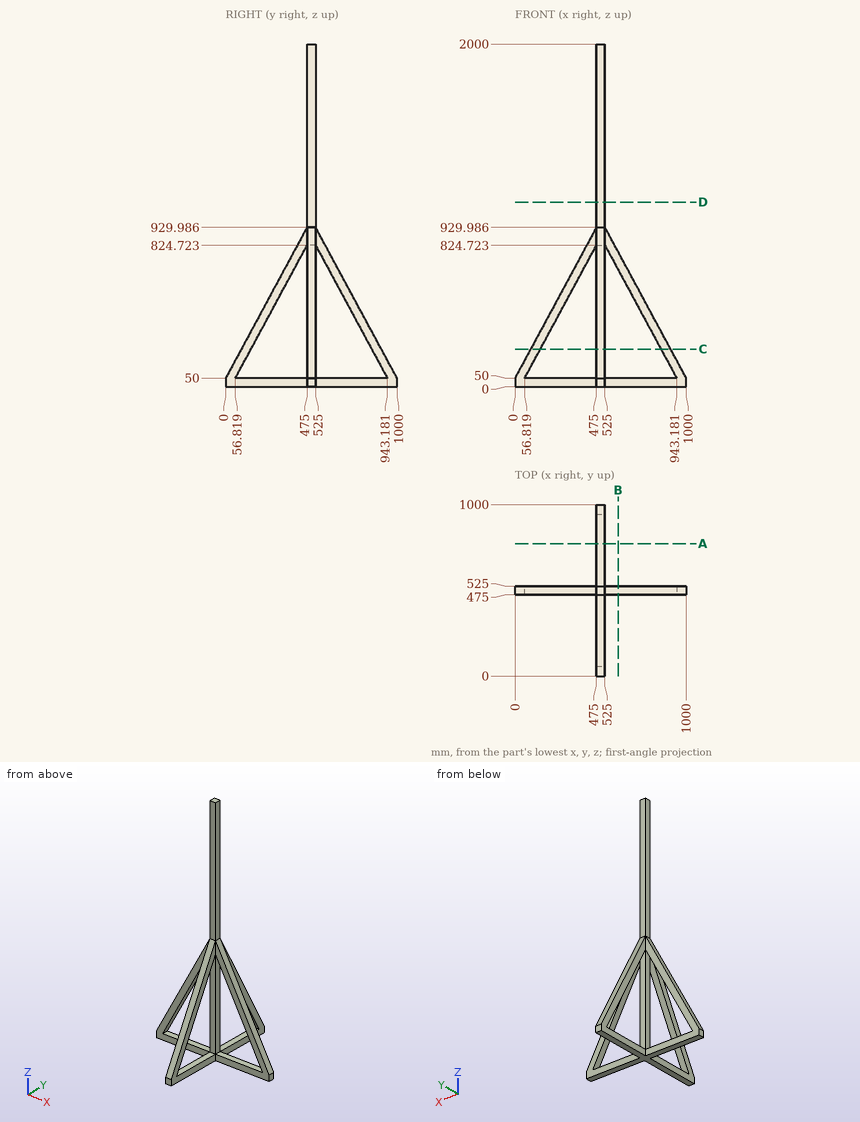
For this review, use the dimensioned drawing (mm, ordinates from the lowest corner) and the shaded views. Coordinates: 2 decimals unless noted, no trailing zeros. Write each loop counter-clockwise with the first axis right and the second up, starting at its lowest first coordinate (ties: lowest second). Pieces come first, ordered by that corner, then holes. Notation, with made-up numbers: (-34, 45.5) - (16, 45.5) arc R28 ccw to (16, 64.5) - close; hole circle Ø11 at (-9, -26.75). An arc over 180 degrees is marked (long way). Answer in a Markdown table with one row per item. Add a question column.
Q1. Consider section D-D on z = 1077.5. Give the boundary of the cut face in (x, y), then the cut area to 3 significant figures.
Q2. Clearance check with flat-ended pins moving along their axes: pin 1 (1 mm diameter, centred on y = 285.5, z = 530.5, fed in from -X); pin 2 (15 mm diameter, centred on x = 508.5, y = 648, fed in from +Z); pin 3 (15 mm diameter, centred on x = 498.5, z = 532, fed in from -Y). State where each tip first meets the part, or that it passes through.
Q3. Consider section C-C on z = 219. Give the boundary of the cut face in (x, y), then the cut area to 3 significant figures.
Q4. Consider section A-A on y = 772. Give the boundary of the cut face in (x, z).
Q5. To check wall thickness, follow line 1 along Y through (x, z) = (647, 693.5); line 2 along Z through (x, y) = (485, 855.5) (1 decimal). State the ranges of each line that lie inside material, in increasing order. Write a range as from..to.
Q6. Consider section B-B on x = 602. Give the boundary of the cut face in (y, z) (1 decimal).
Answers below:
| question | item | result |
|---|---|---|
| 1 | outline | (475, 475) - (525, 475) - (525, 525) - (475, 525) - close |
| 1 | area | 2,500 mm² |
| 2 | pin 1 | x = 475 |
| 2 | pin 2 | z = 716.01 |
| 2 | pin 3 | y = 256.13 |
| 3 | outline | (91.22, 475) - (148.04, 475) - (148.04, 525) - (91.22, 525) - close; (475, 91.22) - (525, 91.22) - (525, 148.04) - (475, 148.04) - close; (475, 475) - (525, 475) - (525, 525) - (475, 525) - close; (475, 851.96) - (525, 851.96) - (525, 908.78) - (475, 908.78) - close; (851.96, 475) - (908.78, 475) - (908.78, 525) - (851.96, 525) - close |
| 3 | area | 13,900 mm² |
| 4 | outline | (475, 0) - (525, 0) - (525, 50) - (475, 50) - close; (475, 367.13) - (525, 367.13) - (525, 472.39) - (475, 472.39) - close |
| 5 | line 1 | 475..525 |
| 5 | line 2 | 0..50, 212.4..317.7 |
| 6 | outline | (475, 0) - (525, 0) - (525, 50) - (475, 50) - close; (475, 682.1) - (525, 682.1) - (525, 787.3) - (475, 787.3) - close |
